Build history of the part. All positions in model axes, mm. Face numbers are marked on the shaded views. A direction names the side the tool comes from. Coordinates: 2 decimals unless noted, no trailing zeros. Order: outer loops, then holes, each group sorted by start corner. A loop starts at its lowest first (then second) coordinate and runs counter-clockwise, first axis right, second up. Notation, with made-up numbers: (78, -2) - (84, -2) arc R36 cw to (84, 33) - close; hole circle Ø11 at (-3.5, 25). An arc over 180 degrees is marked (long way). Write each question's results on one line, items separated by ' | '. Start each with the question number.
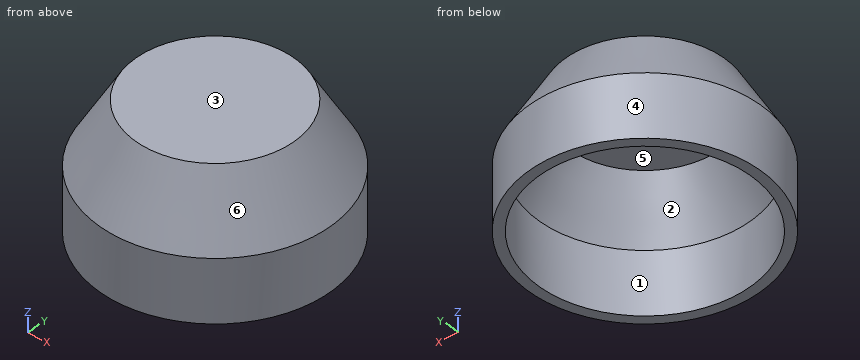
Autodesk Inventor part; units mm, degrees
ref_plane "YZ Plane" through (0, 0, 0) normal (1, 0, 0) x (0, 1, 0)
ref_plane "XZ Plane" through (0, 0, 0) normal (0, 1, 0) x (-1, 0, 0)
ref_plane "XY Plane" through (0, 0, 0) normal (0, 0, 1) x (1, 0, 0)
sketch "Skizze2" plane through (0, 0, 0) normal (0, 1, 0) x (-1, 0, 0)
  line L0 (-60, -3) -> (60, -3)
  line L1 (60, 0) -> (60, -3)
  line L2 (-60, 0) -> (60, 0)
  line L3 (-60, 0) -> (-60, -3)
  line L4 (1.7274, 123.0345) -> (1.7274, -32.1262)
  line L5 (60, 0) -> (60, 31.4988)
  line L6 (60, 31.4988) -> (41.7274, 63.1479)
  line L7 (41.7274, 63.1479) -> (1.7274, 63.1479)
  line L8 (1.7274, 63.1479) -> (1.7274, 58.1479)
  line L9 (39.6141, 58.1479) -> (1.7274, 58.1479)
  line L10 (39.6141, 58.1479) -> (55, 31.4988)
  line L11 (55, 31.4988) -> (55, 0)
  line L12 (60, 0) -> (55, 0)
  point P0 (0, 0)
  dimension "d0" = 31.4988
  dimension "d1" = 150
  dimension "d2" = 40
  dimension "d4" = 31.6491
  dimension "d5" = 150
  dimension "d6" = 5
  dimension "d7" = 5
revolve "Umdrehung1" add sketch "Skizze2" angle 360 about axis through (-1.7274, 0, 123.0345) along (0, 0, -1) contours L2 L11 L10 L9 L4 L7 L6 L5
properties part number "GehaeuseteilB"
Item 1: Slice it at C-C (z = 38.5). Write the cut outline in (x, y).
Item 2: Which spindle directions (+Z, -Z, +X, -X, +Y, -Y) get a long thin tool onto all of the face, cutting with end or side? Do the marked faces 5 and 6. Say none if no direction does.
Item 3: Probe probe 1 along Y at (x, z) = (-43, 21); probe 2 along Z at (x, y) = (-17.5, -23.5); probe 3 along Y at (x, z) = (23, 56). List the from-to ranges inside material, lowest first.
Item 4: Pull direction Y, two halves, no side cores. Call the marked faces 1, 2, 3 and 4: released by +Y, released by -Y, zero draft, split by the parting line, or undercut.
Item 5: Flat gauge pins, fed straight in: P1, Ø2, axis at y = 3, z = 29, coming from the +X side; P2, Ø1, axis at x = -15.5, y = -42, coming from the -Z side; P3, Ø8, axis at x = -40.5, y = -24, coming from the -Z side. Where does each tip first touch, or does it go through?
Item 6: Slice it at A-A (y = 0). Write the cut outline in (x, z).
Item 7: Slice it at B-B (z = 9.5). Write the cut outline in (x, y).
Resolved:
1) outline: circle Ø108.46 at (-1.73, 0); hole circle Ø98.46 at (-1.73, 0)
2) face 5: -Z | face 6: +Z
3) probe 1: -41.14 to -33.68, 33.68 to 41.14 | probe 2: 58.15 to 63.15 | probe 3: -36.55 to -30.32, 30.32 to 36.55
4) face 1: undercut | face 2: undercut | face 3: zero draft | face 4: split by the parting line
5) P1: x = 56.51 | P2: z = 46.35 | P3: z = 37.86
6) outline: (-60, 0) - (-55, 0) - (-55, 31.5) - (-39.61, 58.15) - (36.16, 58.15) - (51.55, 31.5) - (51.55, 0) - (56.55, 0) - (56.55, 31.5) - (38.27, 63.15) - (-41.73, 63.15) - (-60, 31.5) - close
7) outline: circle Ø116.55 at (-1.73, 0); hole circle Ø106.55 at (-1.73, 0)
